```python
from build123d import *

# Parameters (mm, degrees)
BOSS_EXTRU_1_DEPTH           = 3
BOSS_EXTRU_2_START           = -3
ESQUISSE3_R                  = 10
BOSS_EXTRU_2_DEPTH           = 3
CONG_1_R                     = 4
ENL_V_MAT_EXTRU_1_DEPTH      = 48.969384742
ENL_V_MAT_EXTRU_1_DEPTH_BACK = 48.969384742
ESQUISSE2_R                  = 3
ESQUISSE2_R_2                = 2
ENL_V_MAT_EXTRU_2_DEPTH      = 48.969384742
ENL_V_MAT_EXTRU_2_DEPTH_BACK = 48.969384742
ESQUISSE4_R                  = 1.55
ESQUISSE5_R                  = 2.5
ENL_V_MAT_EXTRU_3_DEPTH      = 0.4


with BuildPart() as part:
    # Esquisse1 → Boss.-Extru.1 (new body)
    with BuildSketch(Plane.XY):
        with BuildLine():
            Line((27.916598717, 13.47826087), (20.712315177, 10))
            ThreePointArc((20.712315177, 10), (0, 23), (-20.712315177, 10))
            Line((-20.712315177, 10), (-27.916598717, 13.47826087))
            ThreePointArc((-27.916598717, 13.47826087), (-20.542500679, 23.216495555), (-9.978852639, 29.35))
            ThreePointArc((-9.978852639, 29.35), (0, 40), (9.978852639, 29.35))
            ThreePointArc((9.978852639, 29.35), (20.542500679, 23.216495555), (27.916598717, 13.47826087))
        make_face()
    extrude(amount=BOSS_EXTRU_1_DEPTH)

    # Esquisse3 → Boss.-Extru.2 (add)
    with BuildSketch(Plane.XY.offset(3).offset(BOSS_EXTRU_2_START)):
        with Locations((0, 30)):
            Circle(ESQUISSE3_R)
    extrude(amount=BOSS_EXTRU_2_DEPTH)

    # Congé1
    cong_1_edges = [part.edges().sort_by_distance(p)[0] for p in [
        (-27.916598717, 13.47826087, 1.5),
        (-20.712315177, 10, 1.5),
        (20.712315177, 10, 1.5),
        (27.916598717, 13.47826087, 1.5),
    ]]
    fillet(cong_1_edges, radius=CONG_1_R - 0.0001)  # a hair under: the kernel refuses the full size

    # Esquisse2 → Enlèv. mat.-Extru.1 (cut, two sides: drawn at the far end of the back side and taken through both)
    with BuildSketch(Plane.XY.offset(3).offset(-ENL_V_MAT_EXTRU_1_DEPTH_BACK)):
        with Locations((0, 30)):
            Circle(ESQUISSE2_R)
        with Locations((6, 30)):
            Circle(ESQUISSE2_R_2)
        with Locations((0, 24)):
            Circle(ESQUISSE2_R_2)
        with Locations((-6, 30)):
            Circle(ESQUISSE2_R_2)
        with Locations((0, 36)):
            Circle(ESQUISSE2_R_2)
    extrude(amount=ENL_V_MAT_EXTRU_1_DEPTH + ENL_V_MAT_EXTRU_1_DEPTH_BACK, mode=Mode.SUBTRACT)

    # Esquisse4 → Enlèv. mat.-Extru.2 (cut, two sides: drawn at the far end of the back side and taken through both)
    with BuildSketch(Plane.XY.offset(3).offset(-ENL_V_MAT_EXTRU_2_DEPTH_BACK)):
        with Locations((22.307020844, 15.211733007)):
            Circle(ESQUISSE4_R)
        with Locations((-22.307020844, 15.211733007)):
            Circle(ESQUISSE4_R)
    extrude(amount=ENL_V_MAT_EXTRU_2_DEPTH + ENL_V_MAT_EXTRU_2_DEPTH_BACK, mode=Mode.SUBTRACT)

    # Esquisse5 → Enlèv. mat.-Extru.3 (cut)
    with BuildSketch(Plane.XY.offset(3)):
        with Locations((0, 24)):
            Circle(ESQUISSE5_R)
        with Locations((6, 30)):
            Circle(ESQUISSE5_R)
        with Locations((0, 36)):
            Circle(ESQUISSE5_R)
        with Locations((-6, 30)):
            Circle(ESQUISSE5_R)
    extrude(amount=-ENL_V_MAT_EXTRU_3_DEPTH, mode=Mode.SUBTRACT)


solid = part.part
```
Could you check a few things on this model? Use its own coordinates, in mm. A direction names the side the tool comes from. Round coordinates to 2 decimals unless told otherwise and drop trailing zeros. Loops run counter-clockwise (first coordinate to the right, second up) from the corner with the lowest first, then second, coordinate; pieces in that order, holes last. Notation, with made-up numbers: (57, 43) -> (66, 43) arc R32 cw to (66, 75) -> close; hole circle Ø10 at (-29, 69). An arc over 180 degrees is marked (long way). Put each result on its own line as item: value.
Q1. I want a section at C-C on z = 2.1. Give the number of separate pieces and of enclosed holes in the cut face, and give its area (3 significant figures).
Checks:
separate pieces: 1
enclosed holes: 7
area: 550 mm2
Q2. Please list where these lines run through material, in increasing order: line 1 (Y direction, x = 0, z = 2.7); line 2 (Y direction, x = 0, z = 0.85); line 3 (X direction, y = 30, z = 0.7). Write a range as from..to.
Checks:
line 1: 20..21.5, 26.5..27, 33..33.5, 38.5..40
line 2: 20..22, 26..27, 33..34, 38..40
line 3: -10..-8, -4..-3, 3..4, 8..10
Q3. I want a section at A-A on y = 36. Write out the boundary of the cut face in (x, z), and give its area (3 significant figures).
Checks:
outline: (-8, 0) -> (-2, 0) -> (-2, 2.6) -> (-2.5, 2.6) -> (-2.5, 3) -> (-8, 3) -> close; (2, 0) -> (8, 0) -> (8, 3) -> (2.5, 3) -> (2.5, 2.6) -> (2, 2.6) -> close
area: 35.6 mm2
Q4. I want a section at D-D on y = 24. Write out the boundary of the cut face in (x, z), and give its area (3 significant figures).
Checks:
outline: (-19.62, 0) -> (-2, 0) -> (-2, 2.6) -> (-2.5, 2.6) -> (-2.5, 3) -> (-19.62, 3) -> close; (2, 0) -> (19.62, 0) -> (19.62, 3) -> (2.5, 3) -> (2.5, 2.6) -> (2, 2.6) -> close
area: 105 mm2
Q5. Thinking about a two-plate mould opening in X: for faces 1 (the cylindrical face through (-18.872, 24.593, 1.479)), 2 (the cylindrical face through (26.183, 14.225, 1.521)), 3 (the cylindrical face through (21.31, 11.34, 1.52)), which applies, pulls with the +X half, pulls with the -X half, needs draft (parallel to the pull), parting line crosses it, or undercut?
Checks:
face 1: pulls with the -X half
face 2: pulls with the +X half
face 3: undercut
Q6. Which directions (+Z, -Z, +X, -X, +Y, -Y) give clear straight access to the entire face, cutting with the end or side of a thin tool? Please do faces 4 (the flat face through (5, 32, 2.6)), 5 (the cylindrical face through (-26.16, 14.13, 1.52)), 6 (the cylindrical face through (-13.32, 18.75, 1.48)).
Checks:
face 4: +Z
face 5: +Z, -Z, -X
face 6: +Z, -Z, -Y
Q7. I want a section at B-B on x = 0. Write out the boundary of the cut face in (y, z), and give its area (3 significant figures).
Checks:
outline: (20, 0) -> (22, 0) -> (22, 2.6) -> (21.5, 2.6) -> (21.5, 3) -> (20, 3) -> close; (26, 0) -> (27, 0) -> (27, 3) -> (26.5, 3) -> (26.5, 2.6) -> (26, 2.6) -> close; (33, 0) -> (34, 0) -> (34, 2.6) -> (33.5, 2.6) -> (33.5, 3) -> (33, 3) -> close; (38, 0) -> (40, 0) -> (40, 3) -> (38.5, 3) -> (38.5, 2.6) -> (38, 2.6) -> close
area: 17.2 mm2
Q8. For pin 1 Ø4.5 at (x, y) = (6, 30) entering from +Z, with a flat end and sliding along its axis, tell me the tip position at first contact or that it passes through.
Checks:
pin 1: z = 2.6
